Verification items for the finished model (mm, model axes). A direction names the side the tool comes from. Round coordinates to 2 decimals unless told otherwise and drop trailing zeros. Write each loop counter-clockwise with the first axis right and the second up, starting at its lowest first coordinate (ties: lowest second). Pieces come first, ordered by that corner, then holes. Notation, with made-up numbers: M 64,10 L 104,10 A24 ccw 104,49 Z; hole C 83,11 d11. An arc over 180 degrees is marked long. Answer in a Markdown table with one row per item. Add a question column.
1. Sectioned sample at D-D on y = 56. Record the cut outline in (x, z).
2. Go/stop test with flat-tipped pins: pin 1 Ø1.9 at (x, y) = (2, -30) entering from +Z; pin 2 Ø3 at (x, z) = (3, -40.5) entering from -Y. Record where each tip stops, or that it passes through.
3. Sectioned sample at C-C on z = 37. Record the cut outline in (x, y).
4. Sectioned sample at B-B on y = 28. Record the cut outline in (x, z).
5. Set-up check for faces 1 (the flat face through (3, -27, -31.643)), 2 (the flat face through (3, 66.264, -40)), 3 (the flat face through (6.35, 10, -5)): record each of +Z, -Z, +X, -X, +Y, -Y from which the full face is reachable in a straight line by a thin tool's end or side.
6. Draft check along Z on faces 4 (the cylindrical face through (3.13, 126.05, -43.23)), 5 (the flat face through (3, -16, -50.693)), 6 (the flat face through (3.131, -39.62, 14.125)). Enter one of: pulls with the +Z half, pulls with the -Z half, needs draft (parallel to the pull), parting line crosses it, or undercut.
7. Material ranges on probe 1 along Y at (x, z) = (3.5, -31); probe 2 along Z at (x, y) = (6, 23.5); probe 3 along Z at (x, y) = (4.5, -25.5), recorded low to high.
8. Sectioned sample at A-A on x = 1.5. Record the cut outline in (y, z) (3 decimals).
```python
from build123d import *

# Parameters (mm, degrees)
F0_R     = 1.27
F1_DEPTH = 6.35


with BuildPart() as f1:
    # F0 (on Right) → F1 (new body)
    with BuildSketch(Plane.YZ):
        with BuildLine():
            ThreePointArc((116.750538, -50.692635), (126.088182, -43.047537), (120.436387, -32.384689))
            Line((120.436387, -32.384689), (-93.737434, 57.495441))
            ThreePointArc((-93.737434, 57.495441), (-97.893699, 55.796408), (-99.592732, 59.952673))
            Line((-99.592732, 59.952673), (-110.015241, 64.326581))
            ThreePointArc((-110.015241, 64.326581), (-122.484036, 59.229484), (-117.386939, 46.760689))
            Line((-117.386939, 46.760689), (40.355204, -19.437338))
            ThreePointArc((40.355204, -19.437338), (44.123068, -26.545903), (37.897972, -31.642635))
            Line((37.897972, -31.642635), (-92.790544, -31.642635))
            ThreePointArc((-92.790544, -31.642635), (-102.315544, -41.167635), (-92.790544, -50.692635))
            Line((-92.790544, -50.692635), (63.088998, -50.692635))
            ThreePointArc((63.088998, -50.692635), (65.334062, -49.7627), (66.263998, -47.517635))
            Line((66.263998, -47.517635), (66.263998, -31.642635))
            ThreePointArc((66.263998, -31.642635), (69.438998, -28.467635), (72.613998, -31.642635))
            Line((72.613998, -31.642635), (72.613998, -47.517635))
            ThreePointArc((72.613998, -47.517635), (73.543934, -49.7627), (75.788998, -50.692635))
            Line((75.788998, -50.692635), (116.750538, -50.692635))
        make_face()
        with Locations((108.209478, -36.894451)):
            Circle(F0_R, mode=Mode.SUBTRACT)
        with Locations((97.462779, -32.384689)):
            Circle(F0_R, mode=Mode.SUBTRACT)
        with Locations((108.209478, -36.894451)):
            Circle(F0_R)
        with Locations((97.462779, -32.384689)):
            Circle(F0_R)
    extrude(amount=F1_DEPTH)


solid = f1.part
```
Geometry check:
| question | item | result |
|---|---|---|
| 1 | outline | M 0,-50.69 L 6.35,-50.69 L 6.35,-5.34 L 0,-5.34 Z |
| 2 | pin 1 | stops at z = 31.15 |
| 2 | pin 2 | stops at y = -102.32 |
| 3 | outline | M 0,-94.13 L 6.35,-94.13 L 6.35,-44.9 L 0,-44.9 Z |
| 4 | outline | M 0,-50.69 L 6.35,-50.69 L 6.35,-31.64 L 0,-31.64 Z; M 0,-14.25 L 6.35,-14.25 L 6.35,6.41 L 0,6.41 Z |
| 5 | face 1 | +X, -X, -Y |
| 5 | face 2 | -Z, +X, -X |
| 5 | face 3 | +Z, -Z, +X, +Y, -Y |
| 6 | face 4 | parting line crosses it |
| 6 | face 5 | pulls with the -Z half |
| 6 | face 6 | undercut |
| 7 | probe 1 | y = 40.68 to 66.33, 72.55 to 117.14 |
| 7 | probe 2 | z = -50.69 to -31.64, -12.36 to 8.3 |
| 7 | probe 3 | z = -50.69 to -31.64, 8.2 to 28.86 |
| 8 | outline | M -117.387,46.761 L 40.355,-19.437 A6.35 cw 37.898,-31.643 L -92.791,-31.643 A9.525 ccw -92.791,-50.693 L 63.089,-50.693 A3.175 ccw 66.264,-47.518 L 66.264,-31.643 A3.175 cw 72.614,-31.643 L 72.614,-47.518 A3.175 ccw 75.789,-50.693 L 116.751,-50.693 A9.525 ccw 120.436,-32.385 L -93.737,57.495 A3.175 cw -99.593,59.953 L -110.015,64.327 A9.525 ccw Z |
